Check sheet for the modelled part. Datum: model origin and axes. Units: mm. Coordinates: 2 decimals unless noted, no trailing zeros. Loops run counter-clockwise (first coordinate to the right, second up) from the corner with the lowest first, then second, coordinate; pieces in that order, holes last. Notation, with made-up numbers: (-14.75, 39) -> (28.25, 39) arc R21 cw to (28.25, 64) -> close; hole circle Ø10 at (-21.5, 89). An arc over 180 degrees is marked (long way). Use CSV: the item, a comma, the result in double quotes.
Autodesk Inventor part; units mm, degrees
ref_plane "Work Plane1" through (0, 0, 0) normal (0, 0, 1) x (1, 0, 0)
ref_plane "YZ Plane" through (0, 0, 0) normal (1, 0, 0) x (0, 1, 0)
ref_plane "XZ Plane" through (0, 0, 0) normal (0, 1, 0) x (-1, 0, 0)
sketch "Sketch1" plane through (0, 0, 0) normal (0, 0, 1) x (1, 0, 0)
  arc A0 (10.7315, 12.546514) -> (0, 0) centre (12.7, 0) ccw
  arc A1 (10.7315, 12.546514) -> (0, 0) centre (43.457296, -26.307859) ccw
  dimension "d4" = 12.7
  dimension "d5" = 50.8
  dimension "d6" = 16.51
extrude "Extrusion1" add sketch "Sketch1" against normal blind 355.6
sketch "Sketch2" plane through (0, 0, 0) normal (0, 0, 1) x (1, 0, 0)
  arc A0 (10.7315, 12.546514) -> (0, 0) centre (12.7, 0) ccw
  arc A1 (10.7315, 12.546514) -> (0, 0) centre (43.457296, -26.307859) ccw
  line L0 (3.048836, 8.255) -> (4.852638, 6.712141)
revolve "Revolution1" add sketch "Sketch2" angle 180 about axis through (3.048836, 8.255, 0) along (0.7599342, -0.65, 0) picked at (4.382184, 8.416293) contours A1 L0 A0
sketch "Sketch4" plane through (0, 0, -355.6) normal (0, 0, -1) x (-1, 0, 0)
  arc A0 (0, 0) -> (-10.7315, 12.546514) centre (-12.7, 0) ccw
  arc A1 (0, 0) -> (-10.7315, 12.546514) centre (-43.457296, -26.307859) ccw
  line L0 (-3.048836, 8.255) -> (-4.852638, 6.712141)
revolve "Revolution2" add sketch "Sketch4" angle 180 about axis through (3.048836, 8.255, -355.6) along (0.7599342, -0.65, 0) picked at (-3.096161, 6.912766) contours A1 L0 A0
sketch "Sketch5" plane through (0, 0, 0) normal (0, 0, 1) x (1, 0, 0)
  arc A0 (10.7315, 12.546514) -> (0, 0) centre (43.457296, -26.307859) ccw
  line L0 (0, 0) -> (10.7315, 12.546514)
extrude "Extrusion2" cut sketch "Sketch5" along normal through all both and the other way through all
ref_plane "Work Plane1" through (0, 0, 0) normal (0, 0, 1) x (1, 0, 0)
properties part number "PrimaryHullWireCover" material "Carbon Fiber PLA"
1) Go/stop test with flat-tipped pins: pin 1 Ø1.5 at (x, z) = (4.5, -254) entering from +Y; pin 2 Ø5 at (x, z) = (4.5, -313.5) entering from -Y; pin 3 Ø3 at (x, y) = (6, 8.5) entering from -Z. Record where each tip stops, or that it passes through.
Answer below:
pin 1,"stops at y = 10.29"
pin 2,"stops at y = 3.05"
pin 3,"stops at z = -362.97"
2) Cross-section at C-C on z = -205.5. Record the boundary of the cut face in (x, y).
Answer below:
outline,"(0, 0) arc R50.8 cw to (10.73, 12.55) arc R12.7 ccw to start"
3) Cross-section at B-B on x = 8. Record the boundary of the cut face in (y, z), and give its area (3 significant figures).
Answer below:
outline,"(10.07, -361.75) arc R11.8 ccw to (11.8, -355.6) -> (11.8, 0) arc R11.8 ccw to (10.07, 6.15) -> close"
area,"629 mm²"
4) Cross-section at A-A on y = 10.5. Record the boundary of the cut face in (x, z), and give its area (3 significant figures).
Answer below:
outline,"(5.56, -355.6) arc R7.14 ccw to (8.45, -361.34) -> (8.45, 5.74) arc R7.14 ccw to (5.56, 0) -> close"
area,"1,050 mm²"
5) Thickness scan on line 1 along Y through (x, z) = (10, -318.5); line 2 along X through (y, z) = (9.25, -114); line 3 along X through (y, z) = (8.5, -83). Record the ranges inside material, lowest first. Write a range as from..to.
Answer below:
line 1,"y = 11.92..12.41"
line 2,"x = 4..7.18"
line 3,"x = 3.26..6.46"
